Part model, mm, in its own coordinate system. Face numbers are marked on the shaded views. A direction names the side the tool comes from. Give positions to 0.01 mm unless a question says otherwise; leave off trailing zeros. Order: outer loops, then holes, each group sorted by start corner. A loop starts at its lowest first (then second) coordinate and runs counter-clockwise, first axis right, second up. Notation, with made-up numbers: (62.5, -6) - (100.5, -6) arc R28 ccw to (100.5, 21) - close; hole circle Ø4 at (-27, 32). An arc over 180 degrees is marked (long way). Use one line per item in the form item = value. Start each with the question number.
1. Tool access for the marked faces 1 and 2: list every direction of +Z, -Z, +X, -X, +Y, -Y with a clear straight run to the whole face (end or side of a thin tool).
2. Drill centre lines: line 1 (Y direction, x = 55.35, z = -12.7); line 2 (X direction, y = 12.75, z = -24); line 3 (Y direction, x = 52, z = -13). Where is each one in solid material? Low to high.
3. Band-saw the part on D-D, the plane x = 3.5. List the corners of the cut face in (y, z), plus the area to 3 significant figures.
4. Band-saw the part on A-A, the plane z = -12.7. List the corners of the cut face in (x, y), plus the area to 3 significant figures.
5. Band-saw the part on B-B, the plane y = 11.43. List the corners of the cut face in (x, z), plus the area to 3 significant figures.
6. Band-saw the part on C-C, the plane y = 15.75. List the corners of the cut face in (x, z), plus the area to 3 significant figures.
7. Pull direction X, two halves, no side cores. Call the marked faces 3, 4, 5 and 6: +X half, -X half, draft (parallel to the pull), parting line (faces both ways), or undercut.
8. Pin check, flat tips, straight feed: P1, Ø1.5, axis at x = 21, y = 10.5, coming from the -Z side; P2, Ø7, axis at y = 14, z = -9, coming from the +X side; P3, Ø7, axis at y = 14.5, z = -17.5, coming from the -X side. Stop position of each tip, or through.
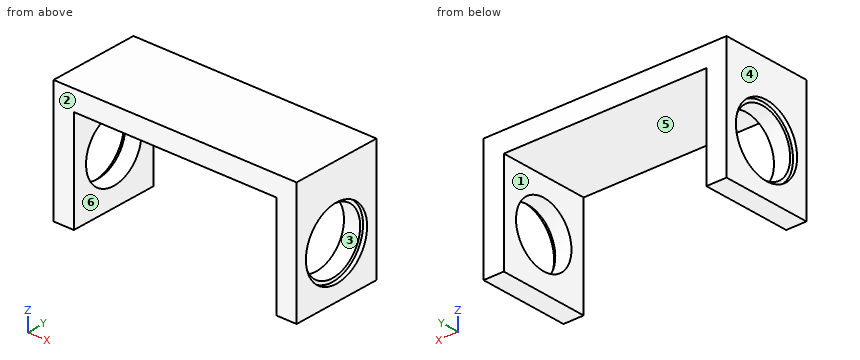
from build123d import *

# Parameters (mm, degrees)
EXTRUDE_THIN1_DEPTH                            = 22.86
CBORE_FOR_6_SOCKET_HEAD_CAP_SCREW1_D           = 15.875
CBORE_FOR_6_SOCKET_HEAD_CAP_SCREW1_DEPTH       = 5.08
CBORE_FOR_6_SOCKET_HEAD_CAP_SCREW1_CBORE_D     = 17.526
CBORE_FOR_6_SOCKET_HEAD_CAP_SCREW1_CBORE_DEPTH = 1.016
CBORE_FOR_6_SOCKET_HEAD_CAP_SCREW2_D           = 15.875
CBORE_FOR_6_SOCKET_HEAD_CAP_SCREW2_CBORE_D     = 17.526
CBORE_FOR_6_SOCKET_HEAD_CAP_SCREW2_CBORE_DEPTH = 1.016


with BuildPart() as part:
    # Sketch1 → Extrude-Thin1 (new body)
    with BuildSketch(Plane(origin=(0, 0, 0), x_dir=(1, 0, 0), z_dir=(0, 1, 0))):
        Polygon((0, 25.4), (0, 0), (50.8, 0), (50.8, 25.4), (55.88, 25.4), (55.88, -5.08), (-5.08, -5.08), (-5.08, 25.4), align=None)
    extrude(amount=EXTRUDE_THIN1_DEPTH)

    # CBORE for #6 Socket Head Cap Screw1
    with Locations(Plane(origin=(55.88, 0, 0), x_dir=(0, 0, -1), z_dir=(1, 0, 0))):
        with Locations((12.7, 11.43)):
            CounterBoreHole(CBORE_FOR_6_SOCKET_HEAD_CAP_SCREW1_D / 2, CBORE_FOR_6_SOCKET_HEAD_CAP_SCREW1_CBORE_D / 2, CBORE_FOR_6_SOCKET_HEAD_CAP_SCREW1_CBORE_DEPTH, depth=CBORE_FOR_6_SOCKET_HEAD_CAP_SCREW1_DEPTH)

    # CBORE for #6 Socket Head Cap Screw2 (through all)
    with Locations(Plane.ZY.offset(5.08)):
        with Locations((-12.7, 11.43)):
            CounterBoreHole(CBORE_FOR_6_SOCKET_HEAD_CAP_SCREW2_D / 2, CBORE_FOR_6_SOCKET_HEAD_CAP_SCREW2_CBORE_D / 2, CBORE_FOR_6_SOCKET_HEAD_CAP_SCREW2_CBORE_DEPTH)


solid = part.part
From the geometry:
q1.face_1 = -Z, +Y, -Y
q1.face_2 = +Z, -Z, +X, -X, -Y
q2.line_1 = 0 to 2.67, 20.19 to 22.86
q2.line_2 = -5.08 to 0, 50.8 to 55.88
q2.line_3 = 0 to 3.5, 19.36 to 22.86
q3.outline = (0, 0) - (22.86, 0) - (22.86, 5.08) - (0, 5.08) - close
q3.area = 116 mm²
q4.outline = (-5.08, 0) - (0, 0) - (0, 3.49) - (-4.06, 3.49) - (-4.06, 2.67) - (-5.08, 2.67) - close; (-5.08, 20.19) - (-4.06, 20.19) - (-4.06, 19.37) - (0, 19.37) - (0, 22.86) - (-5.08, 22.86) - close; (50.8, 0) - (55.88, 0) - (55.88, 2.67) - (54.86, 2.67) - (54.86, 3.49) - (50.8, 3.49) - close; (50.8, 19.37) - (54.86, 19.37) - (54.86, 20.19) - (55.88, 20.19) - (55.88, 22.86) - (50.8, 22.86) - close
q4.area = 67.6 mm²
q5.outline = (-5.08, -25.4) - (0, -25.4) - (0, -20.64) - (-4.06, -20.64) - (-4.06, -21.46) - (-5.08, -21.46) - close; (-5.08, -3.94) - (-4.06, -3.94) - (-4.06, -4.76) - (0, -4.76) - (0, 0) - (50.8, 0) - (50.8, -4.76) - (54.86, -4.76) - (54.86, -3.94) - (55.88, -3.94) - (55.88, 5.08) - (-5.08, 5.08) - close; (50.8, -25.4) - (55.88, -25.4) - (55.88, -21.46) - (54.86, -21.46) - (54.86, -20.64) - (50.8, -20.64) - close
q5.area = 403 mm²
q6.outline = (-5.08, -25.4) - (0, -25.4) - (0, -19.36) - (-4.06, -19.36) - (-4.06, -20.32) - (-5.08, -20.32) - close; (-5.08, -5.08) - (-4.06, -5.08) - (-4.06, -6.04) - (0, -6.04) - (0, 0) - (50.8, 0) - (50.8, -6.04) - (54.86, -6.04) - (54.86, -5.08) - (55.88, -5.08) - (55.88, 5.08) - (-5.08, 5.08) - close; (50.8, -25.4) - (55.88, -25.4) - (55.88, -20.32) - (54.86, -20.32) - (54.86, -19.36) - (50.8, -19.36) - close
q6.area = 429 mm²
q7.face_3 = draft
q7.face_4 = -X half
q7.face_5 = undercut
q7.face_6 = undercut
q8.P1 = 0
q8.P2 = 54.86
q8.P3 = -5.08
